```python
from build123d import *

# Parameters (mm, degrees)
BOSS_EXTRUDE1_DEPTH   = 1500
BOSS_EXTRUDE1_2_DEPTH = 1500
SKETCH5_W             = 460
SKETCH5_H             = 460
BOSS_EXTRUDE5_DEPTH   = 25
SKETCH6_W             = 1500
SKETCH6_H             = 460
BOSS_EXTRUDE6_DEPTH   = 5


with BuildPart() as part:
    # Sketch1 → Boss-Extrude1 (new body)
    with BuildSketch(Plane.XY):
        Polygon((0, -30), (217.5, -30), (217.5, -5), (242.5, -5), (242.5, -30), (460, -30), (460, 0), (0, 0), align=None)
    extrude(amount=BOSS_EXTRUDE1_DEPTH)



with BuildPart() as body_2:
    # Sketch1 → Boss-Extrude1 2 (new body)
    with BuildSketch(Plane.XY):
        Polygon((242.5, -430), (460, -430), (460, -460), (0, -460), (0, -430), (217.5, -430), (217.5, -455), (242.5, -455), align=None)
    extrude(amount=BOSS_EXTRUDE1_2_DEPTH)


with BuildPart() as part_1:
    add(part.part)

    add(body_2.part)  # Boss-Extrude5 merges body 2
    # Sketch5 → Boss-Extrude5 (add)
    with BuildSketch(Plane(origin=(0, 0, 0), x_dir=(-1, 0, 0), z_dir=(0, 0, -1))):
        with Locations((-230, -230)):
            Rectangle(SKETCH5_W, SKETCH5_H)
    extrude(amount=-BOSS_EXTRUDE5_DEPTH)

    # Sketch6 → Boss-Extrude6 (add)
    with BuildSketch(Plane.ZY):
        with Locations((750, -230)):
            Rectangle(SKETCH6_W, SKETCH6_H)
    extrude(amount=BOSS_EXTRUDE6_DEPTH)


solid = part_1.part
```
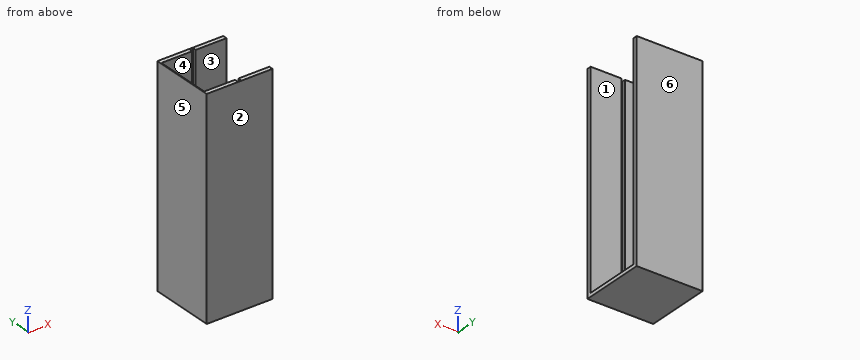
Source: CAD feature listing. Evaluate the final solid. Frame: model axes, mm. Face numbers are marked on the shaded views. A direction names the side the tool comes from. Coordinates: 2 decimals unless noted, no trailing zeros. Write each loop counter-clockwise with the first axis right and the second up, starting at its lowest first coordinate (ties: lowest second). Pieces come first, ordered by that corner, then holes. Notation, with made-up numbers: M -11,8 L 46,8 A24 cw 46,41 Z; hole C -37,82 d3. An arc over 180 degrees is marked long. Answer as a JSON object with one key per item and string values.
1. Contact query for flat-ended pins moving along their axis: P1, Ø3, axis at y = -411.5, z = 181, coming from the +X side; P2, Ø1, axis at x = 294.5, y = -412.5, coming from the +Z side. Output: stop coordinate, or through.
Evaluation:
{"P1": "x = 0", "P2": "z = 25"}
2. Access query for the marked faces 1 and 2. Directions: +Z, -Z, +X, -X, +Y, -Y. A direction counts if a zero-diameter tool reaches every point of the face in a straight line with its end or side. Return the directions, or none.
Evaluation:
{"face 1": "+Z, +X", "face 2": "+Z, -Z, +X, -X, -Y"}
3. Draft query along Y for the marked faces 3, 4, 5 and 6. Return one class per face: released by +Y, released by -Y, zero draft, split by the parting line, or undercut.
Evaluation:
{"face 3": "undercut", "face 4": "undercut", "face 5": "zero draft", "face 6": "released by +Y"}
4. Cut plane A-A on x = 423.5. Output: boundary loops of the cut face in (y, z).
Evaluation:
{"outline": "M -460,0 L 0,0 L 0,1500 L -30,1500 L -30,25 L -430,25 L -430,1500 L -460,1500 Z"}
5. Cut plane C-C on z = 1383. Output: boundary loops of the cut face in (x, y), plus the area to 4 significant figures.
Evaluation:
{"outline": "M -5,-460 L 460,-460 L 460,-430 L 242.5,-430 L 242.5,-455 L 217.5,-455 L 217.5,-430 L 0,-430 L 0,-30 L 217.5,-30 L 217.5,-5 L 242.5,-5 L 242.5,-30 L 460,-30 L 460,0 L -5,0 Z", "area": "28,650 mm^2"}
6. Cut plane B-B on y = -309. Output: boundary loops of the cut face in (x, z).
Evaluation:
{"outline": "M -5,0 L 460,0 L 460,25 L 0,25 L 0,1500 L -5,1500 Z"}
7. Ray query, L1, parallel to Y at x = 306.5, z = 1017; L2, parallel to X at y = -63, z = 743; L3, parallel to Z at x = 252.5, y = -172. Return the intervals inside material, ascending.
Evaluation:
{"L1": "-460 to -430, -30 to 0", "L2": "-5 to 0", "L3": "0 to 25"}
